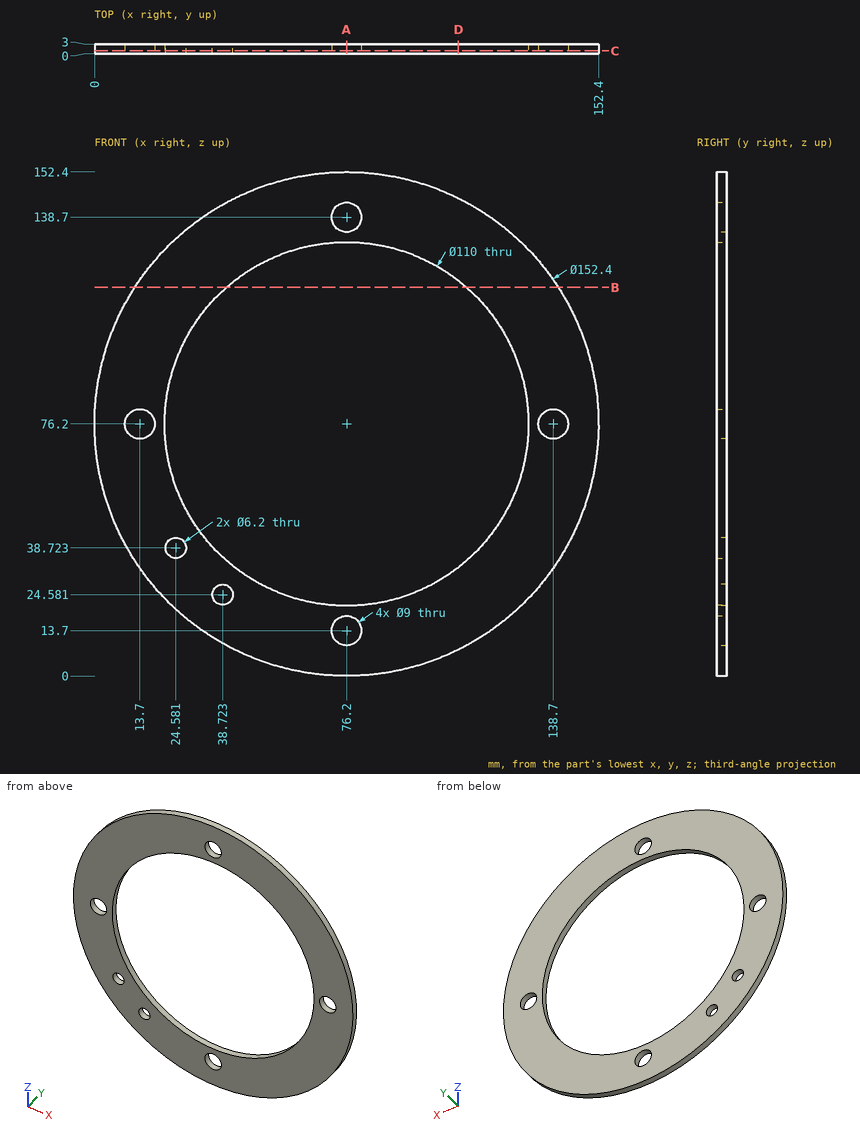
Geometry: see drawing. Coordinates: mm, zero at the bounding-box minimum. Coordinates: 2 decimals unless noted, no trailing zeros. Order: outer loops, then holes, each group sorted by start corner. A loop starts at its lowest first (then second) coordinate and runs counter-clockwise, first axis right, second up. Notation, with made-up numbers: (67.25, 72) - (100.25, 72) arc R30 ccw to (100.25, 108) - close; hole circle Ø5 at (75, 73.5). An arc over 180 degrees is marked (long way). Use one line per item in the form item = value.
1) Section D-D (x = 110). Return loops of the section in (y, z).
Solutions:
outline = (0, 7.91) - (3, 7.91) - (3, 32.81) - (0, 32.81) - close; (0, 119.59) - (3, 119.59) - (3, 144.49) - (0, 144.49) - close
2) Pin query (flat end, axial travel): pin 1 (1.5 mm diameter, centred on y = 0.5, z = 82, fed in from +X); pin 2 (1 mm diameter, centred on x = 133.5, y = 0.5, fed in from +Z) (1 decimal); pin 3 (1.5 mm diameter, centred on y = 2.5, z = 58.5, fed in from +X); pin 4 (10.5 mm diameter, centred on x = 13.7, z = 76.2, fed in from -Y). Return the tip coordinate at first contact, or that it passes through.
Solutions:
pin_1 = 152.23
pin_2 = 127
pin_3 = 150.49
pin_4 = 0
3) Section B-B (z = 117.5). Return loops of the section in (x, y), then the cut area to 3 significant figures.
Solutions:
outline = (12.16, 0) - (39.88, 0) - (39.88, 3) - (12.16, 3) - close; (112.52, 0) - (140.24, 0) - (140.24, 3) - (112.52, 3) - close
area = 166 mm^2
4) Section A-A (x = 76.2). Return loops of the section in (y, z), then the cut area to 3 significant figures.
Solutions:
outline = (0, 0) - (3, 0) - (3, 9.2) - (0, 9.2) - close; (0, 18.2) - (3, 18.2) - (3, 21.2) - (0, 21.2) - close; (0, 131.2) - (3, 131.2) - (3, 134.2) - (0, 134.2) - close; (0, 143.2) - (3, 143.2) - (3, 152.4) - (0, 152.4) - close
area = 73.2 mm^2
5) Section C-C (y = 0.95). Return loops of the section in (x, z), then the cut area to 3 significant figures.
Solutions:
outline = circle Ø152.4 at (76.2, 76.2); hole circle Ø9 at (13.7, 76.2); hole circle Ø110 at (76.2, 76.2); hole circle Ø6.2 at (24.58, 38.72); hole circle Ø6.2 at (38.72, 24.58); hole circle Ø9 at (76.2, 13.7); hole circle Ø9 at (76.2, 138.7); hole circle Ø9 at (138.7, 76.2)
area = 8,420 mm^2
6) Ray query, L1, parallel to X at y = 0.7, z = 72.5 (1 decimal); L2, parallel to Z at x = 40.5, y = 0.1; L3, parallel to Z at x = 61, y = 1.5. Return the intervals inside material, ascending.
Solutions:
L1 = 0.1 to 11.1, 16.3 to 21.3, 131.1 to 136.1, 141.3 to 152.3
L2 = 8.88 to 22.04, 27.12 to 34.36, 118.04 to 143.52
L3 = 1.53 to 23.34, 129.06 to 150.87
